```python
from build123d import *

# Parameters (mm, degrees)
SKETCH2_W          = 9
SKETCH2_H          = 9
CUT_EXTRUDE1_DEPTH = 6


with BuildPart() as part:
    # Sketch1 → Revolve1 (revolve)
    with BuildSketch(Plane.XY, mode=Mode.PRIVATE) as revolve1_sk:
        Polygon((-1, 12), (-6, 12), (-6, 16), (-38, 16), (-38, 18), (-6, 18), (-6, 43), (0, 43), (0, 10), (-1, 10), align=None)
    revolve(revolve1_sk.sketch.rotate(Axis((-42.809570876, 0, 0), (1, 0, 0)), 90), axis=Axis((-42.809570876, 0, 0), (1, 0, 0)))

    # Sketch2 → Cut-Extrude1 (cut)
    with BuildSketch(Plane(origin=(0, 0, 0), x_dir=(0, 0, -1), z_dir=(1, 0, 0))):
        with BuildLine():
            Line((-18, -39.05124838), (-18, 39.05124838))
            ThreePointArc((-18, 39.05124838), (-43, 0), (-18, -39.05124838))
        make_face()
        with Locations((0, 30.5)):
            Rectangle(SKETCH2_W, SKETCH2_H)
        with BuildLine():
            ThreePointArc((43, 0), (36.214637924, 23.184046239), (18, 39.05124838))
            Line((18, 39.05124838), (18, -39.05124838))
            ThreePointArc((18, -39.05124838), (36.214637924, -23.184046239), (43, 0))
        make_face()
    extrude(amount=-CUT_EXTRUDE1_DEPTH, mode=Mode.SUBTRACT)


solid = part.part
```
Model file for the job. Use its own axes, mm. A direction names the side the tool comes from. Coordinates: 2 decimals unless noted, no trailing zeros. Order: outer loops, then holes, each group sorted by start corner. A loop starts at its lowest first (then second) coordinate and runs counter-clockwise, first axis right, second up. Notation, with made-up numbers: (72, 20.5) -> (92, 20.5) arc R29 ccw to (92, 51.5) -> close; hole circle Ø11 at (-5, 5.5). An arc over 180 degrees is marked (long way). Answer as a JSON object with one key per item and string values. Group by question number.
1) Cut at B-B, the plane x = -5. Write the cut outline in (y, z).
2) Cut at A-A, the plane z = 0. Write the cut outline in (x, y), then the cut area to 3 significant figures.
3) Which spindle directions (+Z, -Z, +X, -X, +Y, -Y) get a long thin tool onto all of the face, cutting with end or side? Do faces 5 (the face through (-6, -12, -2)), 6 (the face through (-38, 11, 12)), 7 (the face through (-3, 30, 4.5)). Say none if no direction does.
4) Cut at D-D, the plane x = -27. Write the cut outline in (y, z).
5) Cut at C-C, the plane y = -3. Write the cut outline in (x, z).
6) Flat gauge pins, fed straight in: pin 1 (6 mm diameter, centred on x = -33.5, z = 1, fed in from +Y); pin 2 (1 mm diameter, centred on x = -22, z = 9.5, fed in from -Y); pin 3 (1.8 mm diameter, centred on x = -2, z = 2, fed in from -Y). Where does each tip first touch, or does it go through?
7) Drill centre lines: L1, parallel to Y at x = -4.25, z = 0; L2, parallel to Y at x = -0.4, z = 0; L3, parallel to Y at x = -16, z = 0.5. Where is each one in solid material? Low to high.
8) Pull direction Z, two halves, no side cores. Call faces 1 (the face through (-3, 43, 0)), 2 (the face through (-22.22, 15.62, -3.47)), 3 (the face through (-6, 21, 0)), 4 (the face through (-0.51, -0.44, -9.99)): +Z half, -Z half, draft (parallel to the pull), parting line (faces both ways), or undercut.
Check values:
{
 "1": {"outline": "(-39.05, -18) -> (39.05, -18) arc R43 ccw to (39.05, 18) -> (-39.05, 18) arc R43 ccw to start; hole circle Ø24 at (0, 0); hole (26, -4.5) -> (35, -4.5) -> (35, 4.5) -> (26, 4.5) -> close"},
 "2": {"outline": "(-38, -18) -> (-6, -18) -> (-6, -43) -> (0, -43) -> (0, -10) -> (-1, -10) -> (-1, -12) -> (-6, -12) -> (-6, -16) -> (-38, -16) -> close; (-38, 16) -> (-6, 16) -> (-6, 12) -> (-1, 12) -> (-1, 10) -> (0, 10) -> (0, 26) -> (-6, 26) -> (-6, 18) -> (-38, 18) -> close; (-6, 35) -> (0, 35) -> (0, 43) -> (-6, 43) -> close", "area": "450 mm²"},
 "3": {"face 5": "-X", "face 6": "+Z, -Z, -X, +Y, -Y", "face 7": "+X, -X"},
 "4": {"outline": "circle Ø36 at (0, 0); hole circle Ø32 at (0, 0)"},
 "5": {"outline": "(-38, -17.75) -> (-6, -17.75) -> (-6, -18) -> (0, -18) -> (0, -9.54) -> (-1, -9.54) -> (-1, -11.62) -> (-6, -11.62) -> (-6, -15.72) -> (-38, -15.72) -> close; (-38, 15.72) -> (-6, 15.72) -> (-6, 11.62) -> (-1, 11.62) -> (-1, 9.54) -> (0, 9.54) -> (0, 18) -> (-6, 18) -> (-6, 17.75) -> (-38, 17.75) -> close"},
 "6": {"pin 1": "stops at y = 18", "pin 2": "stops at y = -15.59", "pin 3": "stops at y = -42.99"},
 "7": {"L1": "y = -43 to -12, 12 to 26, 35 to 43", "L2": "y = -43 to -10, 10 to 26, 35 to 43", "L3": "y = -17.99 to -15.99, 15.99 to 17.99"},
 "8": {"face 1": "parting line", "face 2": "undercut", "face 3": "draft", "face 4": "undercut"}
}
